Work out the finished part from the listing and answer in its coordinate system (mm). A direction names the side the tool comes from. Round coordinates to 2 decimals unless told otherwise and drop trailing zeros. Loops run counter-clockwise (first coordinate to the right, second up) from the corner with the lowest first, then second, coordinate; pieces in that order, holes last. Notation, with made-up numbers: (-23.5, 70.25) -> (10.5, 70.25) arc R14 cw to (10.5, 96.25) -> close; hole circle Ø6 at (37, 77.5). An arc over 180 degrees is marked (long way). Use one line per item in the form item = value.
```python
from build123d import *

# Parameters (mm, degrees)
BOSS_EXTRUDE1_DEPTH = 13
SKETCH2_R           = 11
CUT_EXTRUDE1_DEPTH  = 111.390216958
SKETCH3_W           = 32
SKETCH3_H           = 64
BOSS_EXTRUDE2_DEPTH = 45
CUT_EXTRUDE2_DEPTH  = 19


# Read off the part's stored shape, not the designer's step: Mirror1
with BuildPart() as part:
    # Sketch1 → Boss-Extrude1 (new body)
    with BuildSketch(Plane(origin=(0, 0, 0), x_dir=(1, 0, 0), z_dir=(0, 1, 0))):
        with BuildLine():
            ThreePointArc((-57, 64), (-89, 32), (-57, 0))
            Line((-57, 0), (-57, 64))
        make_face()
        with BuildLine():
            Line((-57, 64), (-57, 0))
            ThreePointArc((-57, 0), (-34.372583002, 9.372583002), (-25, 32))
            ThreePointArc((-25, 32), (-34.372583002, 54.627416998), (-57, 64))
        make_face()
        with BuildLine():
            Line((-57, 0), (0, 0))
            Line((0, 0), (0, 64))
            Line((0, 64), (-57, 64))
            ThreePointArc((-57, 64), (-34.372583002, 54.627416998), (-25, 32))
            ThreePointArc((-25, 32), (-34.372583002, 9.372583002), (-57, 0))
        make_face()
    extrude(amount=BOSS_EXTRUDE1_DEPTH)

    # Sketch2 → Cut-Extrude1 (cut, through all)
    with BuildSketch(Plane(origin=(0, 13, 0), x_dir=(1, 0, 0), z_dir=(0, 1, 0))):
        with Locations(Location((-57, 32, 0), (0, 0, 270))):
            Circle(SKETCH2_R)
    extrude(amount=-CUT_EXTRUDE1_DEPTH, mode=Mode.SUBTRACT)

    # Sketch3 → Boss-Extrude2 (add)
    with BuildSketch(Plane(origin=(0, 13, 0), x_dir=(1, 0, 0), z_dir=(0, 1, 0))):
        with Locations((-16, 32)):
            Rectangle(SKETCH3_W, SKETCH3_H)
    extrude(amount=BOSS_EXTRUDE2_DEPTH)

    # Sketch4 → Cut-Extrude2 (cut)
    with BuildSketch(Plane(origin=(0, 0, 0), x_dir=(0, 0, -1), z_dir=(1, 0, 0))):
        Polygon((0, 13), (51, 58), (0, 58), align=None)
    extrude(amount=-CUT_EXTRUDE2_DEPTH, mode=Mode.SUBTRACT)

    # Mirror1: part across plane


with BuildPart() as part_1:
    add(part.part)
    add(part.part.mirror(Plane(origin=(0, 0, 0), x_dir=(0, 0, 1), z_dir=(1, 0, 0))))


solid = part_1.part
```
(1) Given P1, Ø6, axis at y = 24.5, z = -45, coming from the +X side; P2, Ø8, axis at y = 32.5, z = -52, coming from the -X side; P3, Ø3, axis at x = -10.5, z = -27.5, coming from the +Y side, each flat-ended and moving along its own axis, determine where each tip first touches the part or whether it passes through.
Completed:
P1 = 32
P2 = -32
P3 = 38.59
(2) Find section A-A, the plane z = -32. Write down the section's boundary in (x, y), then the cut area to 3 significant figures.
Completed:
outline = (-89, 0) -> (-68, 0) -> (-68, 13) -> (-89, 13) -> close; (-46, 0) -> (46, 0) -> (46, 13) -> (32, 13) -> (32, 58) -> (19, 58) -> (19, 41.24) -> (-19, 41.24) -> (-19, 58) -> (-32, 58) -> (-32, 13) -> (-46, 13) -> close; (68, 0) -> (89, 0) -> (89, 13) -> (68, 13) -> close
area = 3,980 mm2
(3) Consider L1, parallel to X at y = 3.5, z = -32; L2, parallel to Z at x = 57, y = 3; L3, parallel to X at y = 8.5, z = -34. Determine where each line is inside the solid, lowest interval first.
Completed:
L1 = -89 to -68, -46 to 46, 68 to 89
L2 = -64 to -43, -21 to 0
L3 = -88.94 to -67.82, -46.18 to 46.18, 67.82 to 88.94
(4) Find section C-C, the plane y = 35.5. Write down the section's boundary in (x, z), then the cut area to 3 significant figures.
Completed:
outline = (-32, -64) -> (32, -64) -> (32, 0) -> (19, 0) -> (19, -25.5) -> (-19, -25.5) -> (-19, 0) -> (-32, 0) -> close
area = 3,130 mm2
(5) Find section D-D, the plane z = -54. Write down the section's boundary in (x, y).
Completed:
outline = (-80.24, 0) -> (80.24, 0) -> (80.24, 13) -> (32, 13) -> (32, 58) -> (-32, 58) -> (-32, 13) -> (-80.24, 13) -> close
(6) Find section B-B, the plane y = 7. Write down the section's boundary in (x, z).
Completed:
outline = (-57, -64) -> (57, -64) arc R32 ccw to (57, 0) -> (-57, 0) arc R32 ccw to start; hole circle Ø22 at (-57, -32); hole circle Ø22 at (57, -32)
(7) For faces 1 (the flat face through (-67, 13, -25)), 2 (the cylindrical face through (-47.725, 6.591, -26.086)), 3 (the flat face through (67, 13, -25)), 4 (the flat face through (19, 41, -19)), determine the directions among +Z, -Z, +X, -X, +Y, -Y from which every point of the face is accessible in a straight line to the end or side of a thin tool.
Completed:
face_1 = +Z, -Z, -X, +Y
face_2 = +Y, -Y
face_3 = +Z, -Z, +X, +Y
face_4 = +Z, +Y
(8) For a pull along X with two mould halves and no side action, classify faces 5 (the flat face through (-19, 41, -19)), 6 (the flat face through (1, 0, -32)), 7 (the flat face through (-32, 35, -32)) as +X half, -X half, draft (parallel to the pull), parting line (faces both ways), or undercut.
Completed:
face_5 = undercut
face_6 = draft
face_7 = -X half
